Check sheet for the modelled part. Datum: model origin and axes. Units: mm. Coordinates: 2 decimals unless noted, no trailing zeros. Write each loop counter-clockwise with the first axis right and the second up, starting at its lowest first coordinate (ties: lowest second). Pieces come first, ordered by that corner, then holes. Notation, with made-up numbers: (39.5, 37) - (95.5, 37) arc R20 ccw to (95.5, 61) - close; hole circle Ø2 at (1.5, 84). An arc over 180 degrees is marked (long way). Write each question's results on one line, items separated by ' | '.
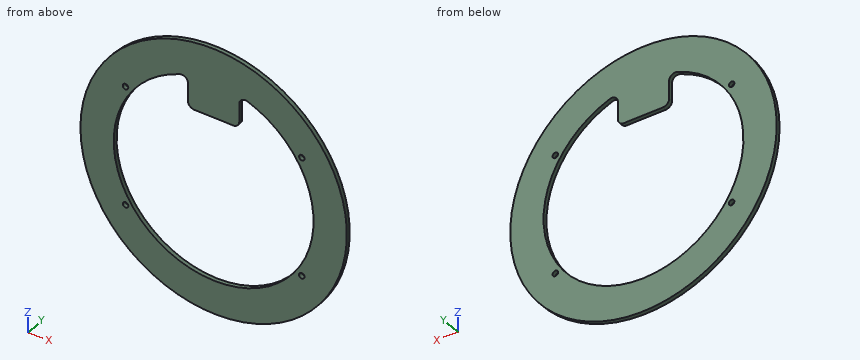
Autodesk Inventor part; units mm, degrees
ref_plane "YZ Plane" through (0, 0, 0) normal (1, 0, 0) x (0, 1, 0)
ref_plane "XZ Plane" through (0, 0, 0) normal (0, 1, 0) x (-1, 0, 0)
ref_plane "XY Plane" through (0, 0, 0) normal (0, 0, 1) x (1, 0, 0)
sketch "Sketch1" plane through (0, 0, 0) normal (0, 1, 0) x (-1, 0, 0)
  circle A0 centre (0, 0) radius 65
  line L0 (0, 0) -> (65, 0) construction
  line L1 (0, 0) -> (0, -65) construction
  circle A1 centre (0, 0) radius 48.75
  line L2 (0, 48.75) -> (0, 31.25)
  line L3 (0, 31.25) -> (-37.4166, 31.25)
  line L4 (0, 31.25) -> (37.4166, 31.25)
  line L5 (0, 0) -> (65, 0) construction
  line L6 (0, 0) -> (-48.75, 0) construction
  circle A2 centre (29, 43) radius 1.35
  circle A3 centre (-29, 43) radius 1.35
  circle A4 centre (29, -43) radius 1.35
  circle A5 centre (-29, -43) radius 1.35
  circle A6 centre (-43, 29) radius 1.35
  circle A7 centre (-43, -29) radius 1.35
  circle A8 centre (43, 29) radius 1.35
  circle A9 centre (43, -29) radius 1.35
  circle A10 centre (-29, -43) radius 1.35
  circle A11 centre (29, -43) radius 1.35
  circle A12 centre (-29, 43) radius 1.35
  circle A13 centre (29, 43) radius 1.35
  circle A14 centre (43, -29) radius 1.35
  circle A15 centre (43, 29) radius 1.35
  circle A16 centre (-43, -29) radius 1.35
  circle A17 centre (-43, 29) radius 1.35
  line L7 (12.5, 48.75) -> (-12.5, 48.75)
  line L8 (-12.5, 48.75) -> (-12.5, 31.25)
  line L9 (-12.5, 31.25) -> (12.5, 31.25)
  line L10 (12.5, 31.25) -> (12.5, 48.75)
  line L11 (12.5, 48.75) -> (-12.5, 31.25) construction
  line L12 (-12.5, 48.75) -> (12.5, 31.25) construction
  point P0 (0, -48.75)
  point P1 (0, 40)
  point P2 (-12.5, 47.1202)
  point P3 (12.5, 47.1202)
  dimension "d0" = 130
  dimension "d18" = 97.5
  dimension "d21" = 62.5
  dimension "d29" = 86
  dimension "d30" = 29
  dimension "d31" = 2.7
  dimension "d47" = 360
  dimension "d49" = 25
extrude "Extrusion1" add sketch "Sketch1" along normal blind 2 contours A0 | L10 L4 L2 A1 | A1 L7 L10 | L8 L7 A1 | A1 L2 L3 L8 | A2 | A3 | A4 | A5
sketch "Sketch2" plane through (0, 0, 0) normal (0, -1, 0) x (1, 0, 0)
  circle A0 centre (0, 0) radius 65 construction
  line L0 (-4, 55) -> (4, 55)
  line L1 (4, 55) -> (4, 61)
  line L2 (-4, 61) -> (-4, 55)
  line L3 (-4, 55) -> (4, 61) construction
  line L4 (4, 55) -> (-4, 61) construction
  line L5 (0, 0) -> (0, 71.2779) construction
  arc A1 (4, 61) -> (-4, 61) centre (0, 61) ccw
  line L6 (-24.7431, 49.2826) -> (-17.3521, 52.3441)
  line L7 (-17.3521, 52.3441) -> (-19.6482, 57.8874)
  line L8 (-27.0392, 54.8259) -> (-24.7431, 49.2826)
  line L9 (-24.7431, 49.2826) -> (-19.6482, 57.8874) construction
  line L10 (-17.3521, 52.3441) -> (-27.0392, 54.8259) construction
  arc A2 (-19.6482, 57.8874) -> (-27.0392, 54.8259) centre (-23.3437, 56.3567) ccw
  line L11 (-41.7193, 36.0624) -> (-36.0624, 41.7193)
  line L12 (-36.0624, 41.7193) -> (-40.3051, 45.9619)
  line L13 (-45.9619, 40.3051) -> (-41.7193, 36.0624)
  line L14 (-41.7193, 36.0624) -> (-40.3051, 45.9619) construction
  line L15 (-36.0624, 41.7193) -> (-45.9619, 40.3051) construction
  arc A3 (-40.3051, 45.9619) -> (-45.9619, 40.3051) centre (-43.1335, 43.1335) ccw
  line L16 (-52.3441, 17.3521) -> (-49.2826, 24.7431)
  line L17 (-49.2826, 24.7431) -> (-54.8259, 27.0392)
  line L18 (-57.8874, 19.6482) -> (-52.3441, 17.3521)
  line L19 (-52.3441, 17.3521) -> (-54.8259, 27.0392) construction
  line L20 (-49.2826, 24.7431) -> (-57.8874, 19.6482) construction
  arc A4 (-54.8259, 27.0392) -> (-57.8874, 19.6482) centre (-56.3567, 23.3437) ccw
  line L21 (-55, -4) -> (-55, 4)
  line L22 (-55, 4) -> (-61, 4)
  line L23 (-61, -4) -> (-55, -4)
  line L24 (-55, -4) -> (-61, 4) construction
  line L25 (-55, 4) -> (-61, -4) construction
  arc A5 (-61, 4) -> (-61, -4) centre (-61, 0) ccw
  line L26 (-49.2826, -24.7431) -> (-52.3441, -17.3521)
  line L27 (-52.3441, -17.3521) -> (-57.8874, -19.6482)
  line L28 (-54.8259, -27.0392) -> (-49.2826, -24.7431)
  line L29 (-49.2826, -24.7431) -> (-57.8874, -19.6482) construction
  line L30 (-52.3441, -17.3521) -> (-54.8259, -27.0392) construction
  arc A6 (-57.8874, -19.6482) -> (-54.8259, -27.0392) centre (-56.3567, -23.3437) ccw
  line L31 (-36.0624, -41.7193) -> (-41.7193, -36.0624)
  line L32 (-41.7193, -36.0624) -> (-45.9619, -40.3051)
  line L33 (-40.3051, -45.9619) -> (-36.0624, -41.7193)
  line L34 (-36.0624, -41.7193) -> (-45.9619, -40.3051) construction
  line L35 (-41.7193, -36.0624) -> (-40.3051, -45.9619) construction
  arc A7 (-45.9619, -40.3051) -> (-40.3051, -45.9619) centre (-43.1335, -43.1335) ccw
  line L36 (-17.3521, -52.3441) -> (-24.7431, -49.2826)
  line L37 (-24.7431, -49.2826) -> (-27.0392, -54.8259)
  line L38 (-19.6482, -57.8874) -> (-17.3521, -52.3441)
  line L39 (-17.3521, -52.3441) -> (-27.0392, -54.8259) construction
  line L40 (-24.7431, -49.2826) -> (-19.6482, -57.8874) construction
  arc A8 (-27.0392, -54.8259) -> (-19.6482, -57.8874) centre (-23.3437, -56.3567) ccw
  line L41 (4, -55) -> (-4, -55)
  line L42 (-4, -55) -> (-4, -61)
  line L43 (4, -61) -> (4, -55)
  line L44 (4, -55) -> (-4, -61) construction
  line L45 (-4, -55) -> (4, -61) construction
  arc A9 (-4, -61) -> (4, -61) centre (0, -61) ccw
  line L46 (24.7431, -49.2826) -> (17.3521, -52.3441)
  line L47 (17.3521, -52.3441) -> (19.6482, -57.8874)
  line L48 (27.0392, -54.8259) -> (24.7431, -49.2826)
  line L49 (24.7431, -49.2826) -> (19.6482, -57.8874) construction
  line L50 (17.3521, -52.3441) -> (27.0392, -54.8259) construction
  arc A10 (19.6482, -57.8874) -> (27.0392, -54.8259) centre (23.3437, -56.3567) ccw
  line L51 (41.7193, -36.0624) -> (36.0624, -41.7193)
  line L52 (36.0624, -41.7193) -> (40.3051, -45.9619)
  line L53 (45.9619, -40.3051) -> (41.7193, -36.0624)
  line L54 (41.7193, -36.0624) -> (40.3051, -45.9619) construction
  line L55 (36.0624, -41.7193) -> (45.9619, -40.3051) construction
  arc A11 (40.3051, -45.9619) -> (45.9619, -40.3051) centre (43.1335, -43.1335) ccw
  line L56 (52.3441, -17.3521) -> (49.2826, -24.7431)
  line L57 (49.2826, -24.7431) -> (54.8259, -27.0392)
  line L58 (57.8874, -19.6482) -> (52.3441, -17.3521)
  line L59 (52.3441, -17.3521) -> (54.8259, -27.0392) construction
  line L60 (49.2826, -24.7431) -> (57.8874, -19.6482) construction
  arc A12 (54.8259, -27.0392) -> (57.8874, -19.6482) centre (56.3567, -23.3437) ccw
  line L61 (55, 4) -> (55, -4)
  line L62 (55, -4) -> (61, -4)
  line L63 (61, 4) -> (55, 4)
  line L64 (55, 4) -> (61, -4) construction
  line L65 (55, -4) -> (61, 4) construction
  arc A13 (61, -4) -> (61, 4) centre (61, 0) ccw
  line L66 (49.2826, 24.7431) -> (52.3441, 17.3521)
  line L67 (52.3441, 17.3521) -> (57.8874, 19.6482)
  line L68 (54.8259, 27.0392) -> (49.2826, 24.7431)
  line L69 (49.2826, 24.7431) -> (57.8874, 19.6482) construction
  line L70 (52.3441, 17.3521) -> (54.8259, 27.0392) construction
  arc A14 (57.8874, 19.6482) -> (54.8259, 27.0392) centre (56.3567, 23.3437) ccw
  line L71 (36.0624, 41.7193) -> (41.7193, 36.0624)
  line L72 (41.7193, 36.0624) -> (45.9619, 40.3051)
  line L73 (40.3051, 45.9619) -> (36.0624, 41.7193)
  line L74 (36.0624, 41.7193) -> (45.9619, 40.3051) construction
  line L75 (41.7193, 36.0624) -> (40.3051, 45.9619) construction
  arc A15 (45.9619, 40.3051) -> (40.3051, 45.9619) centre (43.1335, 43.1335) ccw
  line L76 (17.3521, 52.3441) -> (24.7431, 49.2826)
  line L77 (24.7431, 49.2826) -> (27.0392, 54.8259)
  line L78 (19.6482, 57.8874) -> (17.3521, 52.3441)
  line L79 (17.3521, 52.3441) -> (27.0392, 54.8259) construction
  line L80 (24.7431, 49.2826) -> (19.6482, 57.8874) construction
  arc A16 (27.0392, 54.8259) -> (19.6482, 57.8874) centre (23.3437, 56.3567) ccw
  point P0 (0, 58)
  point P1 (-22.1956, 53.585)
  point P2 (-41.0122, 41.0122)
  point P3 (-53.585, 22.1956)
  point P4 (-58, 0)
  point P5 (-53.585, -22.1956)
  point P6 (-41.0122, -41.0122)
  point P7 (-22.1956, -53.585)
  point P8 (0, -58)
  point P9 (22.1956, -53.585)
  point P10 (41.0122, -41.0122)
  point P11 (53.585, -22.1956)
  point P12 (58, 0)
  point P13 (53.585, 22.1956)
  point P14 (41.0122, 41.0122)
  point P15 (22.1956, 53.585)
  dimension "d34" = 8
  dimension "d35" = 6
  dimension "d38" = 4
  dimension "d39" = 55
  dimension "d42" = 360
extrude "Extrusion2" [suppressed]
fillet "Fillet1" radius 3 4 edges at (12.5, 1, 47.1202) (12.5, 1, 31.25) (-12.5, 1, 31.25) (-12.5, 1, 47.1202)
properties part number "IR Board"
1. Go/stop test with flat-tipped pins: pin 1 (2 mm diameter, centred on x = -43, z = -29, fed in from -Y); pin 2 (1 mm diameter, centred on y = 1.5, z = 28, fed in from +X); pin 3 (1.5 mm diameter, centred on x = 29.5, z = -40.5, fed in from -Y). Record where each tip stops, or that it passes through.
Values follow:
pin 1: passes through | pin 2: stops at x = 58.9 | pin 3: stops at y = 0
2. Sectioned sample at D-D (z = 41). Record the cut outline in (x, y), then the cut area to 3 significant figures.
Values follow:
outline: (-50.44, 0) - (-26.37, 0) - (-26.37, 2) - (-50.44, 2) - close; (-12.5, 0) - (12.5, 0) - (12.5, 2) - (-12.5, 2) - close; (26.37, 0) - (50.44, 0) - (50.44, 2) - (26.37, 2) - close | area: 146 mm^2
3. Sectioned sample at A-A (x = 0). Record the cut outline in (y, z), then the cut area to 3 significant figures.
Values follow:
outline: (0, -65) - (2, -65) - (2, -48.75) - (0, -48.75) - close; (0, 31.25) - (2, 31.25) - (2, 65) - (0, 65) - close | area: 100 mm^2
4. Material ranges on L1, parallel to Z at x = -43, y = 1.5; L2, parallel to X at y = 0.85, z = 1; L3, parallel to X at y = 1.6, z = -44.5, recorded low to high. Write a range as [from, to].
Values follow:
L1: z = [-48.74, -30.35], [-27.65, -22.97], [22.97, 27.65], [30.35, 48.74] | L2: x = [-64.99, -48.74], [48.74, 64.99] | L3: x = [-47.38, -19.91], [19.91, 47.38]
5. Sectioned sample at B-B (y = 0.6). Record the cut outline in (x, z), then the cut area to 3 significant figures.
Values follow:
outline: circle Ø130 at (0, 0); hole circle Ø2.7 at (-43, -29); hole circle Ø2.7 at (-43, 29); hole (-16.52, 45.87) arc R48.75 ccw (long way) to (16.52, 45.87) arc R3 ccw to (12.5, 43.04) - (12.5, 34.25) arc R3 cw to (9.5, 31.25) - (-9.5, 31.25) arc R3 cw to (-12.5, 34.25) - (-12.5, 43.04) arc R3 ccw to start; hole circle Ø2.7 at (43, -29); hole circle Ø2.7 at (43, 29) | area: 6,210 mm^2
6. Sectioned sample at C-C (z = 0). Record the cut outline in (x, y).
Values follow:
outline: (-65, 0) - (-48.75, 0) - (-48.75, 2) - (-65, 2) - close; (48.75, 0) - (65, 0) - (65, 2) - (48.75, 2) - close
